```python
from build123d import *

# Parameters (mm, degrees)
SALIENTE_EXTRUIR1_DEPTH = 9
REDONDEO1_R             = 3
REDONDEO2_R             = 1.5
CROQUIS3_R              = 0.75
CORTAR_EXTRUIR1_DEPTH   = 9
REDONDEO3_R             = 1


with BuildPart() as part:
    # Croquis2 → Saliente-Extruir1 (new body)
    with BuildSketch(Plane.XY):
        Polygon((10, 0), (17, 0), (17, 2), (12, 2), (12, 14), (-2, 14), (-2, 2), (-7, 2), (-7, 0), (0, 0), (0, 12), (10, 12), align=None)
    extrude(amount=SALIENTE_EXTRUIR1_DEPTH)

    # Redondeo1
    redondeo1_edges = [part.edges().sort_by_distance(p)[0] for p in [
        (-7, 1, 0),
        (17, 1, 0),
        (17, 1, 9),
        (-7, 1, 9),
    ]]
    fillet(redondeo1_edges, radius=REDONDEO1_R)

    # Redondeo2
    redondeo2_edges = [part.edges().sort_by_distance(p)[0] for p in [
        (-2, 14, 4.5),
        (12, 14, 4.5),
    ]]
    fillet(redondeo2_edges, radius=REDONDEO2_R)

    # Croquis3 → Cortar-Extruir1 (cut)
    with BuildSketch(Plane(origin=(0, 2, 0), x_dir=(1, 0, 0), z_dir=(0, 1, 0))):
        with Locations(Location((-4.5, -4.5, 0), (0, 0, 270))):
            Circle(CROQUIS3_R)
        with Locations(Location((14.5, -4.5, 0), (0, 0, 270))):
            Circle(CROQUIS3_R)
    extrude(amount=-CORTAR_EXTRUIR1_DEPTH, mode=Mode.SUBTRACT)

    # Redondeo3
    redondeo3_edges = [part.edges().sort_by_distance(p)[0] for p in [
        (-2, 2, 4.5),
        (12, 2, 4.5),
    ]]
    fillet(redondeo3_edges, radius=REDONDEO3_R)


solid = part.part
```
Here's how the part is built. I have some questions about the finished solid (model axes, mm). A direction names the side the tool comes from. Round coordinates to 2 decimals unless told otherwise and drop trailing zeros. Order: outer loops, then holes, each group sorted by start corner. A loop starts at its lowest first (then second) coordinate and runs counter-clockwise, first axis right, second up. Notation, with made-up numbers: M -28.5,82.5 L -22.5,82.5 A4 cw -22.5,87.5 Z; hole C 38,39.5 d8. An arc over 180 degrees is marked long. One line per question, with ' | ' between items.
1) For pin 1 Ø4.5 at (x, z) = (-4.5, 2.5) entering from +Y; pin 2 Ø1.2 at (x, z) = (15.5, 2.5) entering from +Y; pin 3 Ø2.5 at (x, z) = (5, 6) entering from -Y, each with a flat end and sliding along its axis, tell me the tip position at first contact or that it passes through.
Working result:
pin 1: y = 2.34 | pin 2: y = 2 | pin 3: y = 12
2) I need wall thicknesses on line 1 along X through (y, z) = (0.4, 4.5); line 2 along X through (y, z) = (8.5, 1.75); line 3 along X through (y, z) = (0.5, 2). Which ranges of each line are inside material? Lowest first, please.
Working result:
line 1: -7 to -5.25, -3.75 to 0, 10 to 13.75, 15.25 to 17 | line 2: -2 to 0, 10 to 12 | line 3: -6.83 to 0, 10 to 16.83
3) I want a section at D-D, the plane x = 14.5. Write out the boundary of the cut face in (y, z), then the cut area to 3 significant figures.
Working result:
outline: M 0,0.04 L 2,0.04 L 2,3.75 L 0,3.75 Z; M 0,5.25 L 2,5.25 L 2,8.96 L 0,8.96 Z | area: 14.8 mm²
4) For faces 1 (the face through (-2, 8, 4)), 2 (the face through (12, 8, 4)), 3 (the face through (16.14, 1.01, 0.9)), 4 (the face through (0, 6, 4)), which set-ups out of +Z, -Z, +X, -X, +Y, -Y let a thin tool reach every point of the face, with its end or its side?
Working result:
face 1: +Z, -Z, -X, +Y | face 2: +Z, -Z, +X, +Y | face 3: -Z, +X, +Y, -Y | face 4: +Z, -Z, -Y
5) I want a section at C-C, the plane y = 6.25. Write out the boundary of the cut face in (x, z), then the cut area to 3 significant figures.
Working result:
outline: M -2,0 L 0,0 L 0,9 L -2,9 Z; M 10,0 L 12,0 L 12,9 L 10,9 Z | area: 36.0 mm²
6) I want a section at B-B, the plane z = 4.5. Write out the boundary of the cut face in (x, y), then the cut area to 3 significant figures.
Working result:
outline: M -7,0 L -5.25,0 L -5.25,2 L -7,2 Z; M -3.75,0 L 0,0 L 0,12 L 10,12 L 10,0 L 13.75,0 L 13.75,2 L 13,2 A1 cw 12,3 L 12,12.5 A1.5 ccw 10.5,14 L -0.5,14 A1.5 ccw -2,12.5 L -2,3 A1 cw -3,2 L -3.75,2 Z; M 15.25,0 L 17,0 L 17,2 L 15.25,2 Z | area: 89.5 mm²
7) If we mould it in two halves opening along Z, with no side actions, what happens to faces 5 (the face through (-5.232, 1.014, 4.337)), 6 (the face through (15.5, 2, 4.4)), 7 (the face through (5, 12.2, 0))? For each: +Z half, -Z half, draft (parallel to the pull), parting line (faces both ways), or undercut.
Working result:
face 5: undercut | face 6: draft | face 7: -Z half
8) I want a section at A-A, the plane y = 1.75. Write out the boundary of the cut face in (x, z), then the cut area to 3 significant figures.
Working result:
outline: M -7,3 A3 ccw -4,0 L 0,0 L 0,9 L -4,9 A3 ccw -7,6 Z; M 10,0 L 14,0 A3 ccw 17,3 L 17,6 A3 ccw 14,9 L 10,9 Z; hole C -4.5,4.5 d1.5; hole C 14.5,4.5 d1.5 | area: 115 mm²
